from build123d import *

# Parameters (mm, degrees)
THICKEN2_OUTLINE_W   = 62.738
THICKEN2_OUTLINE_H   = 91.567
THICKEN2_OUTLINE_W_2 = 57.658
THICKEN2_OUTLINE_H_2 = 86.487
THICKEN2_DEPTH       = 25.4
THICKEN2_2_OUTLINE_W = 57.658
THICKEN2_2_OUTLINE_H = 86.487
THICKEN2_2_DEPTH     = 2.54
THICKEN2_START       = 22.86
THICKEN2_3_OUTLINE_W = 57.658
THICKEN2_3_OUTLINE_H = 86.487
THICKEN2_3_DEPTH     = 2.54
CHAMFER2_SIZE        = 3.175
SKETCH10_W           = 56.529750703
SKETCH10_H           = 12.7
CUT_EXTRUDE2_DEPTH   = 7.62
CUT_EXTRUDE3_REACH   = 104.516
SKETCH11_W           = 4.318
SKETCH11_H           = 21.59


# Read off the part's stored shape, not the designer's step: Thicken2
with BuildPart() as part:
    # Thicken2 outline → Thicken2 (new body)
    with BuildSketch(Plane.YZ):
        with Locations((7.10118863, 45.7835)):
            Rectangle(THICKEN2_OUTLINE_W, THICKEN2_OUTLINE_H)
        with Locations((7.10118863, 45.7835)):
            Rectangle(THICKEN2_OUTLINE_W_2, THICKEN2_OUTLINE_H_2, mode=Mode.SUBTRACT)
    extrude(amount=THICKEN2_DEPTH)

    # Thicken2 2 outline → Thicken2 2 (add)
    with BuildSketch(Plane.YZ):
        with Locations((7.10118863, 45.7835)):
            Rectangle(THICKEN2_2_OUTLINE_W, THICKEN2_2_OUTLINE_H)
    extrude(amount=THICKEN2_2_DEPTH)

    # Thicken2 3 outline → Thicken2 3 (add)
    with BuildSketch(Plane.YZ.offset(THICKEN2_START)):
        with Locations((7.10118863, 45.7835)):
            Rectangle(THICKEN2_3_OUTLINE_W, THICKEN2_3_OUTLINE_H)
    extrude(amount=THICKEN2_3_DEPTH)

    # Chamfer2
    chamfer2_edges = [part.edges().sort_by_distance(p)[0] for p in [
        (12.7, 38.47018863, 0),
        (12.7, 38.47018863, 91.567),
        (12.7, -24.26781137, 0),
        (12.7, -24.26781137, 91.567),
    ]]
    chamfer(chamfer2_edges, length=CHAMFER2_SIZE)

    # Sketch10 → Cut-Extrude2 (cut)
    with BuildSketch(Plane(origin=(25.4, 0, 0), x_dir=(0, 0, -1), z_dir=(1, 0, 0))):
        with Locations((-12.375124648, -17.91781137)):
            Rectangle(SKETCH10_W, SKETCH10_H)
    extrude(amount=-CUT_EXTRUDE2_DEPTH, mode=Mode.SUBTRACT)

    # Sketch11 → Cut-Extrude3 (cut, up to next)
    with BuildSketch(Plane(origin=(25.4, 0, 0), x_dir=(0, 0, -1), z_dir=(1, 0, 0)), mode=Mode.PRIVATE) as cut_extrude3_sk1:
        with Locations((-62.738, 23.86518863)):
            Rectangle(SKETCH11_W, SKETCH11_H)
    cut_extrude3_tool1 = extrude(cut_extrude3_sk1.sketch, amount=-CUT_EXTRUDE3_REACH, mode=Mode.PRIVATE) & part.part
    add(cut_extrude3_tool1.solids().sort_by_distance((25.4, 23.865189, 62.738))[0], mode=Mode.SUBTRACT)


solid = part.part
Work out the finished part from the listing and answer in its coordinate system (mm). A direction names the side the tool comes from. Round coordinates to 2 decimals unless told otherwise and drop trailing zeros. Order: outer loops, then holes, each group sorted by start corner. A loop starts at its lowest first (then second) coordinate and runs counter-clockwise, first axis right, second up. Notation, with made-up numbers: M -28,66.25 L -24,66.25 A16 ccw -24,74.25 Z; hole C 31.25,16.25 d6. An arc over 180 degrees is marked long. One line per item, written item: value.
Q1. Find section D-D on y = -13. Write down the section's boundary in (x, z).
Derived:
outline: M 0,0 L 17.78,0 L 17.78,2.54 L 2.54,2.54 L 2.54,89.03 L 22.86,89.03 L 22.86,40.64 L 25.4,40.64 L 25.4,91.57 L 0,91.57 Z
Q2. A flat-ended cylindrical pin translates along its axis: pin 1 (8.5 mm diameter, centred on x = 23, y = -20, fed in from -Z). Find the tip coordinate at first contact, or state that the pin passes through.
Derived:
pin 1: z = 40.64
Q3. For faces 4 (the face through (13, 7, 2.54)), 5 (the face through (17.78, -22, 16)), 6 (the face through (25.4, 7, 46)), 7 (the face through (0, 7, 46)), 8 (the face through (24, 24, 60.579)), determine the directions among +Z, -Z, +X, -X, +Y, -Y from which every point of the face is accessible in a straight line to the end or side of a thin tool.
Derived:
face 4: none
face 5: -Z, +X, -Y
face 6: +Z, -Z, +X, +Y, -Y
face 7: +Z, -Z, -X, +Y, -Y
face 8: +X
Q4. Find section A-A on x = 10.25. Write down the section's boundary in (y, z) (3 decimals).
Derived:
outline: M -24.268,3.175 L -21.093,0 L 35.295,0 L 38.47,3.175 L 38.47,88.392 L 35.295,91.567 L -21.093,91.567 L -24.268,88.392 Z; hole M -21.728,2.54 L 35.93,2.54 L 35.93,89.027 L -21.728,89.027 Z
Q5. Find section B-B on z = 50. Write down the section's boundary in (x, y).
Derived:
outline: M 0,-24.27 L 25.4,-24.27 L 25.4,38.47 L 0,38.47 Z; hole M 2.54,-21.73 L 22.86,-21.73 L 22.86,35.93 L 2.54,35.93 Z
Q6. Find section C-C on y = 11. Write down the section's boundary in (x, z), then the cut area to 3 significant figures.
Derived:
outline: M 0,0 L 25.4,0 L 25.4,91.57 L 0,91.57 Z; hole M 2.54,2.54 L 22.86,2.54 L 22.86,89.03 L 2.54,89.03 Z
area: 568 mm²
Q7. Determine the mould class of faces 1 (the face through (24, 24, 64.897)), 2 (the face through (23.3, -19.4, 40.64)), 3 (the face through (12.522, 36.905, 1.61)) for opening direction Y: released by +Y, released by -Y, zero draft, split by the parting line, or undercut.
Derived:
face 1: undercut
face 2: zero draft
face 3: released by +Y
Q8. Straight lines are drawn through the part: line 1 (Y direction, x = 15.75, z = 83.5); line 2 (Z direction, x = 4.5, y = 34); line 3 (X direction, y = 26.5, z = 28.5). For each, find the intervals that lie inside material, in ascending order.
Derived:
line 1: -24.27 to -21.73, 35.93 to 38.47
line 2: 0 to 2.54, 89.03 to 91.57
line 3: 0 to 2.54, 22.86 to 25.4
